Part print with two shaded views. Sizes in mm from the minimum x, y, z corner. Give positions to 0.01 mm unless a question says otherwise; leave off trailing zeros. Write each loop counter-clockwise with the first axis right and the second up, starting at its lowest first coordinate (ties: lowest second). Pieces come first, ordered by that corner, then holes.
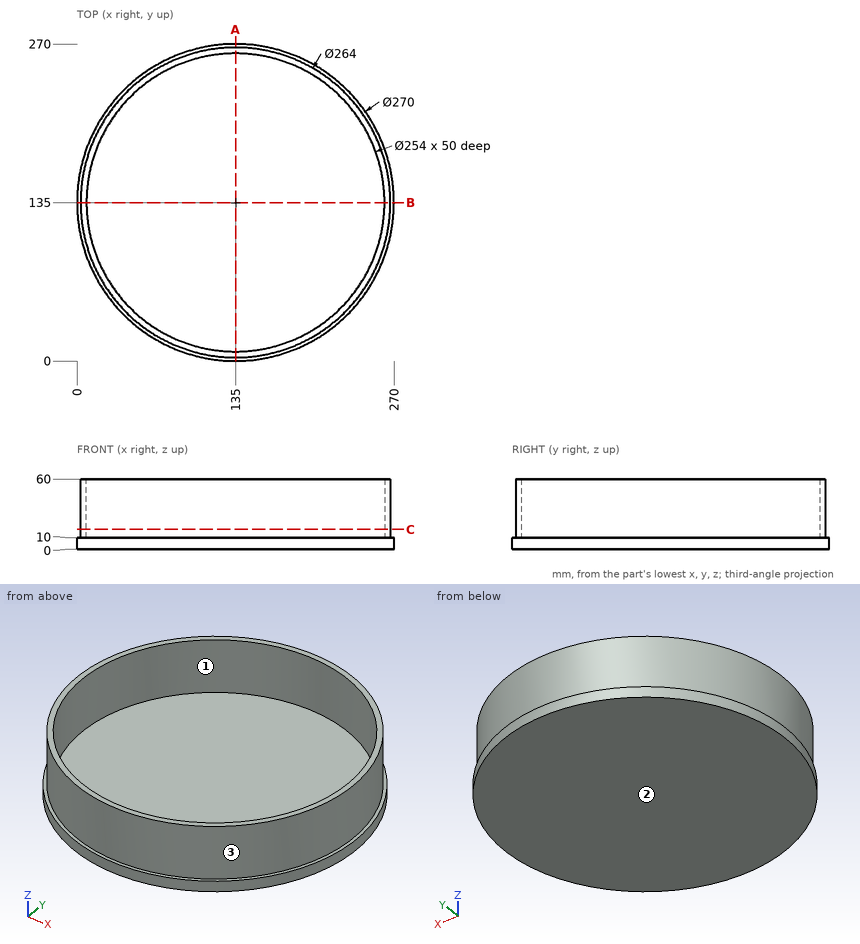
1) Two-plate mould, pull along X, no slides. Class the marked faces 1, 2 and 3: +X half, -X half, draft (parallel to the pull), parting line (faces both ways), or undercut.
Answers follow:
face 1: undercut
face 2: draft
face 3: parting line
2) Wall check: L1, parallel to Y at x = 135, z = 48.5; L2, parallel to Z at x = 87, y = 26; L3, parallel to X at y = 155.5, z = 37. Give the ranges that are in metal, low to high.
Answers follow:
L1: y = 3 to 8, 262 to 267
L2: z = 0 to 10
L3: x = 4.6 to 9.67, 260.33 to 265.4
3) Saw through at A-A, the plane x = 135. Write the cut outline in (y, z).
Answers follow:
outline: (0, 0) - (270, 0) - (270, 10) - (267, 10) - (267, 60) - (262, 60) - (262, 10) - (8, 10) - (8, 60) - (3, 60) - (3, 10) - (0, 10) - close
4) Pin check, flat tips, straight feed: pin 1 Ø2 at (y, z) = (186, 13.5) entering from -X; pin 2 Ø1 at (x, z) = (91.5, 21) entering from -Y; pin 3 Ø3 at (x, y) = (205.5, 78) entering from -Z; pin 4 Ø12 at (x, z) = (196, 7.5) entering from +Y. Stop position of each tip, or through.
Answers follow:
pin 1: stops at x = 12.84
pin 2: stops at y = 10.2
pin 3: stops at z = 0
pin 4: stops at y = 258.29
5) Saw through at C-C, the plane z = 17. Write the cut outline in (x, y).
Answers follow:
outline: circle Ø264 at (135, 135); hole circle Ø254 at (135, 135)
